The listing builds one solid part. Answer for the finished solid, in the listing's coordinates (mm). A direction names the side the tool comes from. Give positions to 0.01 mm unless a question says otherwise; leave off trailing zeros. Order: outer loops, then holes, each group sorted by start corner. A loop starts at its lowest first (then second) coordinate and runs counter-clockwise, first axis right, second up. Notation, with made-up numbers: (83, -34.5) - (126, -34.5) arc R14 ccw to (126, -27.5) - close; hole circle Ø3 at (55.5, -21). An arc over 180 degrees is marked (long way). Write each question's results on one line, items separated by ' | '. Start each with the question number.
1. Find the intervals of material crossed by L1, parallel to Z at x = 50.8, y = -6.5; L2, parallel to Z at x = 50.8, y = -21; L3, parallel to Y at x = 46, z = 7, in increasing order.
2. Section A-A (y = -16.75) is taken. Give the vertices of the cut face in (x, z), and give its area (4 significant figures).
3. Which of the six approach directions +Z, -Z, +X, -X, +Y, -Y give full straight-line access (tool end or side, diameter ignored) to faces 5 (the face through (61, 0, 56)), 6 (the face through (64, -12.7, 24))?
4. Section D-D (y = -11.25) is taken. Give the vertices of the cut face in (x, z).
5. Section C-C (x = 50.8) is taken. Give the vertices of the cut face in (y, z), and give its area (3 significant figures).
6. A flat-ended cylindrical pin translates along its axis: pin 1 (10 mm diameter, centred on x = 53.5, z = 16, fed in from -Y). Find the tip coordinate at first contact, or state that the pin passes through.
7. Section B-B (z = 38.1) is taken. Give the vertices of the cut face in (x, y).
8. Determine the mould class of faces 1 (the face through (50, -13, 0)), 2 (the face through (35.68, -6.26, 26.51)), 3 (the face through (43.917, -18.961, 7.105)), 4 (the face through (0, -13, 38)) for opening direction Z: released by +Z, released by -Z, zero draft, split by the parting line, or undercut.
from build123d import *

# Parameters (mm, degrees)
F0_W     = 101.6
F0_H     = 76.2
F0_R     = 31.75
F1_DEPTH = 25.4
F0_R_2   = 19.05
F2_DEPTH = 12.7


with BuildPart() as f1:
    # F0 (on Front) → F1 (new body)
    with BuildSketch(Plane.XZ):
        with Locations((50.8, 38.1)):
            Rectangle(F0_W, F0_H)
        with Locations((50.8, 38.1)):
            Circle(F0_R, mode=Mode.SUBTRACT)
    extrude(amount=F1_DEPTH)

    # F0 (on Front) → F2 (join)
    with BuildSketch(Plane.XZ):
        with Locations((50.8, 38.1)):
            Circle(F0_R)
        with Locations((50.8, 38.1)):
            Circle(F0_R_2, mode=Mode.SUBTRACT)
    extrude(amount=F2_DEPTH)


solid = f1.part
Reported:
1) L1: 0 to 19.05, 57.15 to 76.2 | L2: 0 to 6.35, 69.85 to 76.2 | L3: -12.7 to 0
2) outline: (0, 0) - (101.6, 0) - (101.6, 76.2) - (0, 76.2) - close; hole circle Ø63.5 at (50.8, 38.1) | area: 4,575 mm²
3) face 5: +Z, -Z, +X, -X, +Y | face 6: -Y
4) outline: (0, 0) - (101.6, 0) - (101.6, 76.2) - (0, 76.2) - close; hole circle Ø38.1 at (50.8, 38.1)
5) outline: (-25.4, 0) - (0, 0) - (0, 19.05) - (-12.7, 19.05) - (-12.7, 6.35) - (-25.4, 6.35) - close; (-25.4, 69.85) - (-12.7, 69.85) - (-12.7, 57.15) - (0, 57.15) - (0, 76.2) - (-25.4, 76.2) - close | area: 645 mm²
6) pin 1: y = -12.7
7) outline: (0, -25.4) - (19.05, -25.4) - (19.05, -12.7) - (31.75, -12.7) - (31.75, 0) - (0, 0) - close; (69.85, -12.7) - (82.55, -12.7) - (82.55, -25.4) - (101.6, -25.4) - (101.6, 0) - (69.85, 0) - close
8) face 1: released by -Z | face 2: undercut | face 3: undercut | face 4: zero draft
